from build123d import *

# Parameters (mm, degrees)
F0_R     = 2.5
F1_DEPTH = 10
F2_SIZE  = 0.5


# Not quite as in the source:
# - a feature names something its author has since deleted; it is built from what else it names


with BuildPart() as f1:
    # F0 (on Front) → F1 (new body)
    with BuildSketch(Plane.XZ):
        with BuildLine():
            Line((0.5, 14), (0.5, 9.9874921777))
            ThreePointArc((0.5, 9.9874921777), (7.2456883731, 6.892024376), (10, 0))
            ThreePointArc((10, 0), (8.100925873, -5.8630196998), (3.125, -9.499177596))
            Line((3.125, -9.499177596), (17.5625, -4.749588798))
            ThreePointArc((17.5625, -4.749588798), (11, 0), (17.5625, 4.749588798))
            Line((17.5625, 4.749588798), (9.375, 7.4430785492))
            ThreePointArc((9.375, 7.4430785492), (8.3798148254, 8.1703101285), (8, 9.3429140684))
            Line((8, 9.3429140684), (8, 13))
            ThreePointArc((8, 13), (7.7071067812, 13.7071067812), (7, 14))
            Line((7, 14), (0.5, 14))
        make_face()
        with BuildLine():
            ThreePointArc((17.5625, 4.749588798), (11, 0), (17.5625, -4.749588798))
            ThreePointArc((17.5625, -4.749588798), (20.0504629365, -2.9315098499), (21, 0))
            ThreePointArc((21, 0), (20.0504629365, 2.9315098499), (17.5625, 4.749588798))
        make_face()
        with Locations((16, 0)):
            Circle(F0_R, mode=Mode.SUBTRACT)
        with BuildLine():
            ThreePointArc((-3.125, -9.499177596), (-9.9104859097, 1.3350164915), (-0.5, 9.9874921777))
            Line((-0.5, 9.9874921777), (-0.5, 14))
            Line((-0.5, 14), (-7, 14))
            ThreePointArc((-7, 14), (-7.7071067812, 13.7071067812), (-8, 13))
            Line((-8, 13), (-8, 9.3429140684))
            ThreePointArc((-8, 9.3429140684), (-8.3798148254, 8.1703101285), (-9.375, 7.4430785492))
            Line((-9.375, 7.4430785492), (-17.5625, 4.749588798))
            ThreePointArc((-17.5625, 4.749588798), (-13.0684901501, 4.0504629365), (-11, 0))
            ThreePointArc((-11, 0), (-13.0684901501, -4.0504629365), (-17.5625, -4.749588798))
            Line((-17.5625, -4.749588798), (-3.125, -9.499177596))
        make_face()
        with BuildLine():
            ThreePointArc((-17.5625, 4.749588798), (-21, 0), (-17.5625, -4.749588798))
            ThreePointArc((-17.5625, -4.749588798), (-13.0684901501, -4.0504629365), (-11, 0))
            ThreePointArc((-11, 0), (-13.0684901501, 4.0504629365), (-17.5625, 4.749588798))
        make_face()
        with Locations((-16, 0)):
            Circle(F0_R, mode=Mode.SUBTRACT)
        with BuildLine():
            ThreePointArc((0.5, 3.9686269666), (3, 2.6457513111), (4, 0))
            ThreePointArc((4, 0), (-2.6457513111, -3), (-0.5, 3.9686269666))
            Line((-0.5, 3.9686269666), (-0.5, 9.9874921777))
            ThreePointArc((-0.5, 9.9874921777), (-9.9104859097, 1.3350164915), (-3.125, -9.499177596))
            ThreePointArc((-3.125, -9.499177596), (0, -10), (3.125, -9.499177596))
            ThreePointArc((3.125, -9.499177596), (8.100925873, -5.8630196998), (10, 0))
            ThreePointArc((10, 0), (7.2456883731, 6.892024376), (0.5, 9.9874921777))
            Line((0.5, 9.9874921777), (0.5, 3.9686269666))
        make_face()
    extrude(amount=F1_DEPTH)

    # F2
    f2_edges = [f1.edges().sort_by_distance(p)[0] for p in [
        (-18.5, -10, 0),
        (0, -10, -4),
        (13.5, -10, 0),
        (13.5, 0, 0),
        (0, 0, -4),
        (-18.5, 0, 0),
    ]]
    chamfer(f2_edges, length=F2_SIZE)


solid = f1.part
The listing builds one solid part. Answer for the finished solid, in the listing's coordinates (mm). A direction names the side the tool comes from. Give positions to 0.01 mm unless a question says otherwise; leave off trailing zeros. Order: outer loops, then holes, each group sorted by start corner. A loop starts at its lowest first (then second) coordinate and runs counter-clockwise, first axis right, second up. Notation, with made-up numbers: (22, 52) - (28, 52) arc R9 ccw to (28, 61) - close; hole circle Ø4 at (-20, 49). An arc over 180 degrees is marked (long way). Answer as CSV lines item,"result".
Q1. Which of the six approach directions +Z, -Z, +X, -X, +Y, -Y give full straight-line access (tool end or side, diameter ignored) to faces 1 (the face through (-8, -5, 11)), 2 (the face through (-4, -5, 14))?
Answer key:
face 1,"+Z, -X, +Y, -Y"
face 2,"+Z, +X, -X, +Y, -Y"
Q2. Each of these flat-tipped pins is pushed along its axis until it touches: pin 1 Ø2 at (y, z) = (-5, -5) entering from +X; pin 2 Ø7 at (x, z) = (0, 0) entering from -Y; pin 3 Ø5 at (x, y) = (-15.5, -6.5) entering from +Z; pin 4 Ø3 at (y, z) = (-4, 10.5) entering from +X. Where does it stop, or does it pass through?
Answer key:
pin 1,"stops at x = 19"
pin 2,"passes through"
pin 3,"stops at z = 6.25"
pin 4,"stops at x = 8.03"
Q3. Determine the mould class of faces 3 (the face through (13.5, -4.9, 0.1)), 4 (the face through (-21, -5, 0)), 5 (the face through (8, -5, 11)) for opening direction Z: pulls with the +Z half, pulls with the -Z half, needs draft (parallel to the pull), parting line crosses it, or undercut.
Answer key:
face 3,"undercut"
face 4,"parting line crosses it"
face 5,"needs draft"
Q4. A cutting plane is placed at B-B, the plane x = 16. Determine the outline of the cut face in (y, z), and give its area (3 significant figures).
Answer key:
outline,"(-10, -5.26) - (0, -5.26) - (0, -3) - (-0.5, -2.5) - (-9.5, -2.5) - (-10, -3) - close; (-10, 3) - (-9.5, 2.5) - (-0.5, 2.5) - (0, 3) - (0, 5.26) - (-10, 5.26) - close"
area,"54.8 mm^2"
Q5. A cutting plane is placed at C-C, the plane x = 0. Determine the outline of the cut face in (y, z).
Answer key:
outline,"(-10, -10) - (0, -10) - (0, -4.5) - (-0.5, -4) - (-9.5, -4) - (-10, -4.5) - close"
Q6. Straight lines are drawn through the part: L1, parallel to X at y = -4.75, z = 13; L2, parallel to X at y = -8, z = 0.25; L3, parallel to X at y = -2.5, z = 0.75. For each, find the intervals that lie inside material, in ascending order.
Answer key:
L1,"x = -8 to -0.5, 0.5 to 8"
L2,"x = -20.99 to -18.49, -13.51 to -3.99, 3.99 to 13.51, 18.49 to 20.99"
L3,"x = -20.94 to -18.38, -13.62 to -3.93, 3.93 to 13.62, 18.38 to 20.94"
Q7. A cutting plane is placed at A-A, the plane y = -1.75. Determine the outline of the cut face in (x, z) (1 decimal), and give its area (3 significant figures).
Answer key:
outline,"(-17.6, -4.7) - (-3.1, -9.5) arc R10 ccw to (3.1, -9.5) - (17.6, -4.7) arc R5 ccw to (17.6, 4.7) - (9.4, 7.4) arc R2 cw to (8, 9.3) - (8, 13) arc R1 ccw to (7, 14) - (0.5, 14) - (0.5, 4) arc R4 cw (long way) to (-0.5, 4) - (-0.5, 14) - (-7, 14) arc R1 ccw to (-8, 13) - (-8, 9.3) arc R2 cw to (-9.4, 7.4) - (-17.6, 4.7) arc R5 ccw to start; hole circle Ø5 at (-16, 0); hole circle Ø5 at (16, 0)"
area,"561 mm^2"
